```python
from build123d import *

# Parameters (mm, degrees)
SKETCH_W        = 31.75
SKETCH_H        = 31.75
SKETCH_W_2      = 26.2128
SKETCH_H_2      = 26.2128
PAD_DEPTH       = 1124.5
POCKET_DEPTH    = 31.75
POCKET001_DEPTH = 31.75


with BuildPart() as part:
    # Sketch → Pad (new body)
    with BuildSketch(Plane.XZ):
        Rectangle(SKETCH_W, SKETCH_H)
        Rectangle(SKETCH_W_2, SKETCH_H_2, mode=Mode.SUBTRACT)
    extrude(amount=PAD_DEPTH)

    # Sketch001 → Pocket (cut)
    with BuildSketch(Plane(origin=(0, 0, 15.875), x_dir=(-1, 0, 0), z_dir=(0, 0, 1))):
        Polygon((15.875, 0), (-15.875, 0), (15.875, 10.583303), align=None)
    extrude(amount=-POCKET_DEPTH, mode=Mode.SUBTRACT)

    # Sketch002 → Pocket001 (cut)
    with BuildSketch(Plane(origin=(0, 0, 15.875), x_dir=(-1, 0, 0), z_dir=(0, 0, 1))):
        Polygon((-15.875, 1124.5), (15.875, 1124.5), (15.875, 1101.615832), align=None)
    extrude(amount=-POCKET001_DEPTH, mode=Mode.SUBTRACT)


solid = part.part
```
Input: part model. Units: mm. Frame: model coordinates. A direction names the side the tool comes from. Round coordinates to 2 decimals unless told otherwise and drop trailing zeros. Loops run counter-clockwise (first coordinate to the right, second up) from the corner with the lowest first, then second, coordinate; pieces in that order, holes last. Notation, with made-up numbers: (82, 85) - (141, 85) arc R28 cw to (141, 122) - close; hole circle Ø10 at (54, 48.25). An arc over 180 degrees is marked (long way). One line per item, written item: value. Start each with the question number.
(1) Ray query, line 1 (Z direction, x = -11, y = -1076.5) (3 decimals); line 2 (Y direction, x = -14, z = -10). Return the intervals inside material, ascending. Write a range as [from, to].
(2) Draft query along X for faces 1 (the flat face through (0, -554, 13.106)), 2 (the flat face through (0, -554, 15.875)), 3 (the flat face through (-0.22, -1112.9, -13.89)). Return one class per face: +X half, -X half, draft (parallel to the pull), parting line (faces both ways), or undercut.
(3) Contact query for flat-ended pins moving along their axis: P1, Ø12, axis at x = 7, z = -1.5, coming from the -Y side; P2, Ø10, axis at x = -7.5, z = -8.5, coming from the +Y side. Output: stop coordinate, or through.
(4) Section C-C, the plane y = -91. Return loops of the section in (x, z) (3 decimals), plus the area to 3 significant figures.
(5) Section B-B, the plane x = -1. Return loops of the section in (y, z) (3 decimals).
(6) Section A-A, the plane z = -0.5. Return loops of the section in (x, y) (1 decimal), plus the area to 3 significant figures.
(7) Access query for faces 4 (the flat face through (-13.106, -549, 0)), 5 (the flat face through (0, -554, -15.875)). Directions: +Z, -Z, +X, -X, +Y, -Y. A direction counts if a zero-diameter tool reaches every point of the face in a straight line with its end or side. Return the directions, or none.
Results below:
1. line 1: [-15.875, -13.106], [13.106, 15.875]
1. line 2: [-1102.97, -9.96]
2. face 1: undercut
2. face 2: draft
2. face 3: -X half
3. P1: through
3. P2: y = -7.14
4. outline: (-15.875, -15.875) - (15.875, -15.875) - (15.875, 15.875) - (-15.875, 15.875) - close; hole (-13.106, -13.106) - (13.106, -13.106) - (13.106, 13.106) - (-13.106, 13.106) - close
4. area: 321 mm^2
5. outline: (-1112.337, -15.875) - (-5.625, -15.875) - (-5.625, -13.106) - (-1112.337, -13.106) - close; (-1112.337, 13.106) - (-5.625, 13.106) - (-5.625, 15.875) - (-1112.337, 15.875) - close
6. outline: (-15.9, -1101.6) - (-13.1, -1103.6) - (-13.1, -9.7) - (-15.9, -10.6) - close; (13.1, -1122.5) - (15.9, -1124.5) - (15.9, 0) - (13.1, -0.9) - close
6. area: 6,130 mm^2
7. face 4: +Y, -Y
7. face 5: -Z, +X, -X, +Y, -Y
